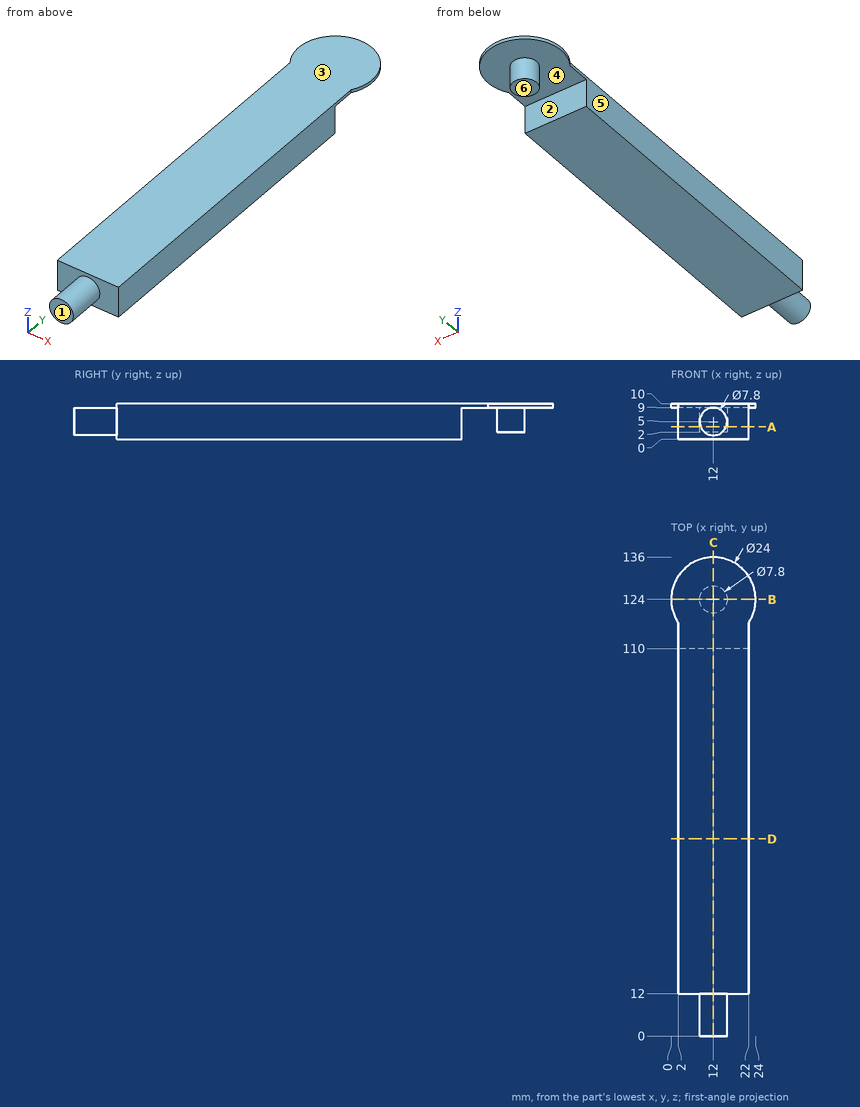
Part print with two shaded views. Sizes in mm from the minimum x, y, z corner. A direction names the side the tool comes from. Round coordinates to 2 decimals unless told otherwise and drop trailing zeros. Loops run counter-clockwise (first coordinate to the right, second up) from the corner with the lowest first, then second, coordinate; pieces in that order, holes last.
1. 3-axis set-ups, long thin cutter, end or side, ignore diameter. For the marked faces 4, 5 and 6: which of +Z, -Z, +X, -X, +Y, -Y reach the whole face in a straight line?
Solutions:
face 4: -Z
face 5: +Z, -Z, -X, -Y
face 6: -Z, +X, -X, +Y
2. Flat gauge pins, fed straight in: pin 1 (2.5 mm diameter, centred on x = 13, y = 125.5, fed in from -Z); pin 2 (3 mm diameter, centred on y = 71.5, z = 3, fed in from +X); pin 3 (1 mm diameter, centred on y = 14.5, z = 2, fed in from -X). Where does each tip first touch, or does it go through?
Solutions:
pin 1: stops at z = 2
pin 2: stops at x = 22
pin 3: stops at x = 2
3. Slice it at B-B (y = 124). Give the cut face in (x, z).
Solutions:
outline: (0, 9) - (8.1, 9) - (8.1, 2) - (15.9, 2) - (15.9, 9) - (24, 9) - (24, 10) - (0, 10) - close
4. Slice it at D-D (y = 56). Give the cut face in (x, z).
Solutions:
outline: (2, 0) - (22, 0) - (22, 10) - (2, 10) - close
5. Slice it at A-A (z = 3.5). Give the cut face in (x, y), and give its area (3 significant figures).
Solutions:
outline: (2, 12) - (8.4, 12) - (8.4, 0) - (15.6, 0) - (15.6, 12) - (22, 12) - (22, 110) - (2, 110) - close; circle Ø7.8 at (12, 124)
area: 2,090 mm2
6. Drill centre lines: line 1 along X through (y, z) = (82, 1.75); line 2 along Y through (x, z) = (7.75, 5.25); line 3 along Y through (x, z) = (9.25, 8.25). Where is each one in solid material? Low to high.
Solutions:
line 1: x = 2 to 22
line 2: y = 12 to 110
line 3: y = 12 to 110, 121.23 to 126.77
7. Two-plate mould, pull along Y, no slides. Class the marked faces 1, 2 and 3: pulls with the +Y half, pulls with the -Y half, needs draft (parallel to the pull), parting line crosses it, or undercut.
Solutions:
face 1: pulls with the -Y half
face 2: undercut
face 3: needs draft
8. Slice it at C-C (x = 12). Give the cut face in (y, z), and give its area (3 significant figures).
Solutions:
outline: (0, 1.1) - (12, 1.1) - (12, 0) - (110, 0) - (110, 9) - (120.1, 9) - (120.1, 2) - (127.9, 2) - (127.9, 9) - (136, 9) - (136, 10) - (12, 10) - (12, 8.9) - (0, 8.9) - close
area: 1,150 mm2
